Can you work these out from the model? Positions are in its coordinate system, mm. A direction names the side the tool comes from. Coordinates: 2 decimals unless noted, no trailing zeros. Loops run counter-clockwise (first coordinate to the right, second up) from the corner with the lowest first, then second, coordinate; pieces in that order, holes last. Notation, with made-up numbers: (-20.5, 63.5) -> (-1.5, 63.5) arc R12 cw to (-1.5, 71.5) -> close; hole circle Ø2 at (87, 1.5). An arc over 180 degrees is marked (long way). Put each result on its own line as item: value. Start each with the question number.
Item 1: For faces 1 (the flat face through (55.208, 34, 2)), 2 (the cylindrical face through (-0.27, 36.47, 2.46)), 3 (the flat face through (41.398, 21, 2)), 4 (the flat face through (53, 37.2, 2)), 5 (the flat face through (53, 4.8, 2)), which set-ups out of +Z, -Z, +X, -X, +Y, -Y let a thin tool reach every point of the face, with its end or its side?
Item 2: Will these pins go through, and if not, where does the flat tip stop? P1, Ø1.5, axis at x = 52, z = 1.5, coming from the +Y side; P2, Ø1.4, axis at x = 48.5, z = 3, coming from the -Y side; P3, Ø2, axis at y = 21, z = 1.5, coming from the +X side.
Item 3: We'd pull the mould along Y, two halves only. Please class faces 6 (the flat face through (-2.17, 1.89, 2.46)), 7 (the flat face through (48, 22.55, 2)), 8 (the cylindrical face through (-0.27, 5.47, 2.46)), 9 (the flat face through (55.208, 8, 2)): pulls with the +Y half, pulls with the -Y half, needs draft (parallel to the pull), parting line crosses it, or undercut.
Item 4: Please list where these lines run through material, in increasing order: L1, parallel to Y at x = 3, z = 3.6; L2, parallel to Y at x = 16.5, z = 0.3; L3, parallel to X at y = 5.5, z = 1.95. Write a range as from..to.
Item 5: If we section it at A-A on y = 21: Please give me the cut outline in (x, z).
Item 6: If we section it at B-B on x = 46: Please give me the cut outline in (y, z).
Item 7: If we section it at D-D on z = 1.85: State how many separate pieces and enclosed holes the cut face has, plus the area to 3 significant figures.
Item 8: If we section it at C-C on y = 36.5: Please give me the cut outline in (x, z), plus the area to 3 significant figures.
Autodesk Inventor part; units mm, degrees
ref_plane "YZ Plane" through (0, 0, 0) normal (1, 0, 0) x (0, 1, 0)
ref_plane "XZ Plane" through (0, 0, 0) normal (0, 1, 0) x (-1, 0, 0)
ref_plane "XY Plane" through (0, 0, 0) normal (0, 0, 1) x (1, 0, 0)
sketch "Boceto1" plane through (0, 0, 0) normal (0, 0, 1) x (1, 0, 0)
  line L0 (1.2797, 34.95) -> (7.0205, 34.95)
  arc A0 (7.0205, 34.95) -> (7.0205, 38.05) centre (7.0205, 36.5) ccw
  line L1 (7.0205, 38.05) -> (1.2797, 38.05)
  arc A1 (1.2797, 38.05) -> (-0.2703, 36.5) centre (1.2797, 36.5) ccw
  arc A2 (-0.2703, 36.5) -> (1.2797, 34.95) centre (1.2797, 36.5) ccw
  line L2 (7.0205, 7.05) -> (1.2797, 7.05)
  arc A3 (1.2797, 7.05) -> (-0.2703, 5.5) centre (1.2797, 5.5) ccw
  arc A4 (-0.2703, 5.5) -> (1.2797, 3.95) centre (1.2797, 5.5) ccw
  line L3 (1.2797, 3.95) -> (7.0205, 3.95)
  arc A5 (7.0205, 3.95) -> (7.0205, 7.05) centre (7.0205, 5.5) ccw
  arc A6 (38.0205, 34.95) -> (38.0205, 38.05) centre (38.0205, 36.5) ccw
  line L4 (38.0205, 38.05) -> (32.2797, 38.05)
  arc A7 (32.2797, 38.05) -> (30.7297, 36.5) centre (32.2797, 36.5) ccw
  arc A8 (30.7297, 36.5) -> (32.2797, 34.95) centre (32.2797, 36.5) ccw
  line L5 (32.2797, 34.95) -> (38.0205, 34.95)
  arc A9 (15.751, 31.95) -> (4.801, 21) centre (15.751, 21) ccw
  arc A10 (4.801, 21) -> (15.751, 10.05) centre (15.751, 21) ccw
  line L6 (15.751, 10.05) -> (21.9491, 10.05)
  arc A11 (21.9491, 10.05) -> (21.9491, 31.95) centre (21.9491, 21) ccw
  line L7 (21.9491, 31.95) -> (15.751, 31.95)
  line L8 (38.0205, 7.05) -> (32.2797, 7.05)
  arc A12 (32.2797, 7.05) -> (30.7297, 5.5) centre (32.2797, 5.5) ccw
  arc A13 (30.7297, 5.5) -> (32.2797, 3.95) centre (32.2797, 5.5) ccw
  line L9 (32.2797, 3.95) -> (38.0205, 3.95)
  arc A14 (38.0205, 3.95) -> (38.0205, 7.05) centre (38.0205, 5.5) ccw
  line L10 (45.2649, -0.2) -> (45.2649, 2.9451)
  line L11 (45.2649, 2.9451) -> (50.2083, 2.9451)
  line L12 (50.2083, 2.9451) -> (50.2083, 4.8)
  line L13 (50.2083, 4.8) -> (55.2083, 4.8)
  line L14 (55.2083, 4.8) -> (55.2083, 11.2)
  line L15 (55.2083, 11.2) -> (50.2083, 11.2)
  line L16 (50.2083, 11.2) -> (50.2083, 19.45)
  line L17 (50.2083, 19.45) -> (45.3976, 19.45)
  line L18 (45.3976, 19.45) -> (45.3976, 18.45)
  line L19 (45.3976, 18.45) -> (43.3976, 18.45)
  line L20 (43.3976, 18.45) -> (43.3976, 19.45)
  line L21 (43.3976, 19.45) -> (41.3976, 19.45)
  line L22 (41.3976, 19.45) -> (41.3976, 22.55)
  line L23 (41.3976, 22.55) -> (43.3976, 22.55)
  line L24 (43.3976, 22.55) -> (43.3976, 23.55)
  line L25 (43.3976, 23.55) -> (45.3976, 23.55)
  line L26 (45.3976, 23.55) -> (45.3976, 22.55)
  line L27 (45.3976, 22.55) -> (50.2083, 22.55)
  line L28 (50.2083, 22.55) -> (50.2083, 30.8)
  line L29 (50.2083, 30.8) -> (55.2083, 30.8)
  line L30 (55.2083, 30.8) -> (55.2083, 37.2)
  line L31 (55.2083, 37.2) -> (50.2083, 37.2)
  line L32 (50.2083, 37.2) -> (50.2083, 42.2)
  line L33 (50.2083, 42.2) -> (-0.0828, 42.2)
  line L34 (-0.0828, 42.2) -> (-4.2, 38.0828)
  line L35 (-4.2, 38.0828) -> (-4.2, 3.9172)
  line L36 (-4.2, 3.9172) -> (-0.0828, -0.2)
  line L37 (-0.0828, -0.2) -> (45.2649, -0.2)
  point P0 (0, 0)
extrude "Extrusión1" add sketch "Boceto1" along normal blind 5
properties part number "carro x lado motor pieza 5 soporte nema"
Solutions:
1. face 1: +Z, -Z, +X, +Y, -Y
1. face 2: +Z, -Z
1. face 3: +Z, -Z, +X
1. face 4: +Z, -Z, +X, +Y
1. face 5: +Z, -Z, +X, -Y
2. P1: y = 37.2
2. P2: y = 2.95
2. P3: x = 41.4
3. face 6: pulls with the -Y half
3. face 7: undercut
3. face 8: undercut
3. face 9: needs draft
4. L1: -0.2..3.95, 7.05..34.95, 38.05..42.2
4. L2: -0.2..10.05, 31.95..42.2
4. L3: -4.2..-0.27, 8.57..30.73, 39.57..55.21
5. outline: (-4.2, 0) -> (4.8, 0) -> (4.8, 5) -> (-4.2, 5) -> close; (32.9, 0) -> (41.4, 0) -> (41.4, 5) -> (32.9, 5) -> close
6. outline: (2.95, 0) -> (19.45, 0) -> (19.45, 5) -> (2.95, 5) -> close; (22.55, 0) -> (42.2, 0) -> (42.2, 5) -> (22.55, 5) -> close
7. separate pieces: 1
7. enclosed holes: 5
7. area: 1,690 mm^2
8. outline: (-4.2, 0) -> (-0.27, 0) -> (-0.27, 5) -> (-4.2, 5) -> close; (8.57, 0) -> (30.73, 0) -> (30.73, 5) -> (8.57, 5) -> close; (39.57, 0) -> (55.21, 0) -> (55.21, 5) -> (39.57, 5) -> close
8. area: 209 mm^2
